```python
from build123d import *

# Parameters (mm, degrees)
CYLINDER_R        = 5
CYLINDER_DEPTH    = 50
BOX_W             = 10
BOX_H             = 10
BOX_DEPTH         = 10
CYLINDER001_R     = 5
CYLINDER001_DEPTH = 100


with BuildPart() as cylinder:
    # Cylinder → Cylinder (new body)
    with BuildSketch(Plane(origin=(5, 5, 10), x_dir=(1, 0, 0), z_dir=(0, 0, 1))):
        Circle(CYLINDER_R)
    extrude(amount=CYLINDER_DEPTH)


with BuildPart() as box:
    # Box → Box (new body)
    with BuildSketch(Plane.XY):
        with Locations((5, 5)):
            Rectangle(BOX_W, BOX_H)
    extrude(amount=BOX_DEPTH)


with BuildPart() as fusion:
    # Cylinder001 → Cylinder001 (new body)
    with BuildSketch(Plane(origin=(5, 5, -100), x_dir=(1, 0, 0), z_dir=(0, 0, 1))):
        Circle(CYLINDER001_R)
    extrude(amount=CYLINDER001_DEPTH)

    # Fusion: union Cylinder, Box
    add(cylinder.part)
    add(box.part)


with BuildPart() as fusion_1:
    # Fusion placement: moved
    add(fusion.part.moved(Location((-5, -5, 0))))


solid = fusion_1.part
```
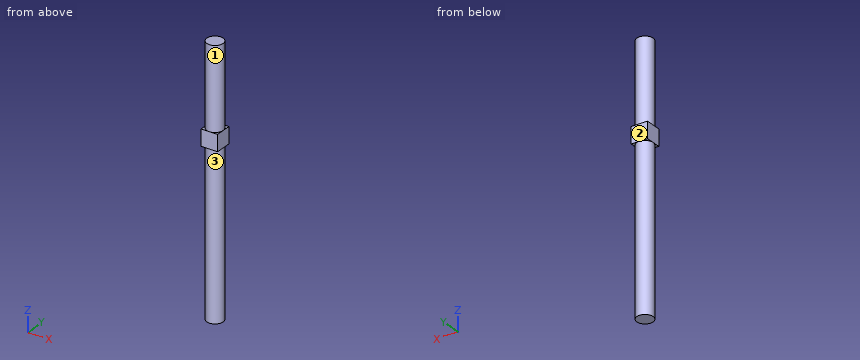
The model under review builds one solid part; all positions refer to its coordinate system, in mm. Face numbers are marked on the shaded views. A direction names the side the tool comes from. Round coordinates to 2 decimals unless told otherwise and drop trailing zeros. Loops run counter-clockwise (first coordinate to the right, second up) from the corner with the lowest first, then second, coordinate; pieces in that order, holes last. Notation, with made-up numbers: (-18, 3.25) -> (34, 3.25) arc R17 ccw to (34, 7.25) -> close; hole circle Ø10 at (-14.75, 35.25). An arc over 180 degrees is marked (long way). Answer as a JSON object with one key per item and string values. Group by question number.
1) We need section B-B on y = -3. Write out the cut boundary in (x, z), then the cut area to 3 significant figures.
2) For the marked faces 1, 2 and 3, list the 3-axis set-ups (+Z, -Z, +X, -X, +Y, -Y) from which the entire face can be reached by the end or side of a thin tool; tool diameter is ignored.
3) We need section A-A on x = -3.5. Write out the cut boundary in (y, z), then the cut area to 3 significant figures.
4) For pin 1 Ø4 at (x, z) = (3, -70) entering from +Y; pin 2 Ø1 at (y, z) = (-2, -16) entering from -X; pin 3 Ø2 at (y, z) = (4, 20) entering from -X, all flat-tipped, find the tip position at first contact; note any pin that passes through.
5) We need section C-C on z = -52.5. Write out the cut boundary in (x, y).
6) For line 1 (X direction, y = -0.25, z = -52.5); line 2 (Y direction, x = 1.25, z = -69.5); line 3 (Z direction, x = -4, y = 3.75), list the stretches that pass through material, from the lowest coordinate up. Write a range as [from, to].
Result set:
{
 "1": {"outline": "(-5, 0) -> (-4, 0) -> (-4, -100) -> (4, -100) -> (4, 0) -> (5, 0) -> (5, 10) -> (4, 10) -> (4, 60) -> (-4, 60) -> (-4, 10) -> (-5, 10) -> close", "area": "1,300 mm²"},
 "2": {"face 1": "+Z", "face 2": "+Z, -Z, +X, -X, +Y", "face 3": "-Z"},
 "3": {"outline": "(-5, 0) -> (-3.57, 0) -> (-3.57, -100) -> (3.57, -100) -> (3.57, 0) -> (5, 0) -> (5, 10) -> (3.57, 10) -> (3.57, 60) -> (-3.57, 60) -> (-3.57, 10) -> (-5, 10) -> close", "area": "1,170 mm²"},
 "4": {"pin 1": "y = 4.9", "pin 2": "x = -4.77", "pin 3": "x = -4"},
 "5": {"outline": "circle Ø10 at (0, 0)"},
 "6": {"line 1": "[-4.99, 4.99]", "line 2": "[-4.84, 4.84]", "line 3": "[0, 10]"}
}
